from build123d import *

# Parameters (mm, degrees)
F0_W     = 119.99976
F0_H     = 125.00102
F1_DEPTH = 10
F2_W     = 12.7
F2_H     = 25.4
F3_DEPTH = 2.54
F4_R     = 6.35
F5_DEPTH = 7.62
F6_R     = 1.27
F7_R     = 2.54
F8_R     = 2.54
F9_DEPTH = 125.00202
F10_R    = 2.54


with BuildPart() as f1:
    # F0 (on Top) → F1 (new body)
    with BuildSketch(Plane.XY):
        Rectangle(F0_W, F0_H)
    extrude(amount=F1_DEPTH)

    # F2 (on face) → F3 (cut)
    with BuildSketch(Plane.XY.offset(10)):
        with Locations((53.64988, -37.59327)):
            Rectangle(F2_W, F2_H)
        Polygon((47.29988, -12.7), (59.99988, -12.7), (59.99988, 12.7), (47.29988, 12.7), (47.29988, 0), align=None)
        with Locations((53.64988, 37.59327)):
            Rectangle(F2_W, F2_H)
    extrude(amount=-F3_DEPTH, mode=Mode.SUBTRACT)

    # F4 (on face) → F5 (join)
    with BuildSketch(Plane.XY.offset(10)):
        with Locations((-40.94988, 0)):
            Circle(F4_R)
        with Locations((-40.94988, -31.24962)):
            Circle(F4_R)
        with Locations((-40.94988, 31.24962)):
            Circle(F4_R)
    extrude(amount=F5_DEPTH)

    # F6
    f6_edges = [f1.edges().sort_by_distance(p)[0] for p in [
        (-47.29988, -31.24962, 17.62),
        (-47.29988, 0, 17.62),
        (-47.29988, 31.24962, 17.62),
    ]]
    fillet(f6_edges, radius=F6_R)

    # F7
    f7_edges = [f1.edges().sort_by_distance(p)[0] for p in [
        (-59.99988, 62.50051, 5),
        (-59.99988, -62.50051, 5),
        (0, 62.50051, 0),
        (-59.99988, 0, 0),
        (0, -62.50051, 0),
        (59.99988, 0, 0),
    ]]
    fillet(f7_edges, radius=F7_R)

    # F8 (on face) → F9 (cut, through all)
    with BuildSketch(Plane.XZ.offset(62.50051)):
        with Locations((59.99988, 10)):
            Circle(F8_R)
    extrude(amount=-F9_DEPTH, mode=Mode.SUBTRACT)

    # F10
    f10_edges = [f1.edges().sort_by_distance(p)[0] for p in [
        (57.45988, 56.39689, 10),
        (57.45988, 18.796635, 10),
        (57.45988, -18.796635, 10),
        (57.45988, -56.39689, 10),
    ]]
    fillet(f10_edges, radius=F10_R)


solid = f1.part
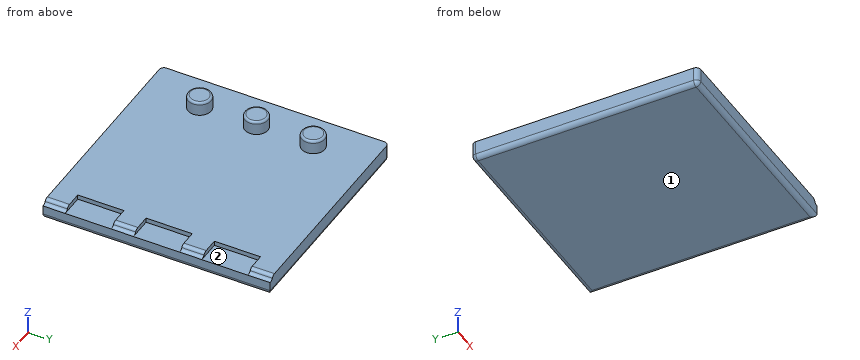
CAD build for the part. Positions are in the model's coordinates, mm. Face numbers are marked on the shaded views. A direction names the side the tool comes from. Coordinates: 2 decimals unless noted, no trailing zeros. Loops run counter-clockwise (first coordinate to the right, second up) from the corner with the lowest first, then second, coordinate; pieces in that order, holes last. Notation, with made-up numbers: (-12, 63.5) -> (-2, 63.5) arc R7 cw to (-2, 69.5) -> close; hole circle Ø1 at (-6.75, 87). An arc over 180 degrees is marked (long way). One line per item, written item: value.
1. Slice it at C-C on z = 14.25. Write the cut outline in (x, y), and give its area (3 significant figures).
Answers:
outline: circle Ø12.7 at (-40.95, -31.25); circle Ø12.7 at (-40.95, 0); circle Ø12.7 at (-40.95, 31.25)
area: 380 mm^2
2. Flat gauge pins, fed straight in: P1, Ø3, axis at y = -3, z = 9, coming from the +X side; P2, Ø6.5, axis at x = 51, y = 32, coming from the +Z side; P3, Ø10, axis at y = 40, z = 15.5, coming from the +X side. Where does each tip first touch, or does it go through?
Answers:
P1: stops at x = 47.3
P2: stops at z = 7.46
P3: stops at x = -35.83
3. Which spindle directions (+Z, -Z, +X, -X, +Y, -Y) get a long thin tool onto all of the face, cutting with end or side? Do the marked faces 1 and 2. Say none if no direction does.
Answers:
face 1: -Z, +X, -X, +Y, -Y
face 2: +Z, +X
4. Drill centre lines: line 1 (X direction, y = -39, z = 7.5); line 2 (Z direction, x = 17.5, y = 0.5); line 3 (X direction, y = 19, z = 2.25). Where is each one in solid material? Low to high. Write a range as [from, to].
Answers:
line 1: x = [-60, 47.3]
line 2: z = [0, 10]
line 3: x = [-59.98, 59.98]
5. Slice it at B-B on y = 53.5. Write the cut outline in (x, z).
Answers:
outline: (-60, 2.54) arc R2.54 ccw to (-57.46, 0) -> (57.46, 0) arc R2.54 ccw to (60, 2.54) -> (60, 7.46) arc R2.54 cw to (57.8, 8.73) arc R2.54 ccw to (55.6, 10) -> (-60, 10) -> close
6. Slice it at D-D on y = 0. Write the cut outline in (x, z), and give its area (3 significant figures).
Answers:
outline: (-60, 2.54) arc R2.54 ccw to (-57.46, 0) -> (57.46, 0) arc R2.54 ccw to (60, 2.54) -> (60, 7.46) -> (47.3, 7.46) -> (47.3, 10) -> (-34.6, 10) -> (-34.6, 16.35) arc R1.27 ccw to (-35.87, 17.62) -> (-46.03, 17.62) arc R1.27 ccw to (-47.3, 16.35) -> (-47.3, 10) -> (-60, 10) -> close
area: 1,260 mm^2
7. Slice it at A-A on x = -24. Write the cut outline in (y, z), and give its area (3 significant figures).
Answers:
outline: (-62.5, 2.54) arc R2.54 ccw to (-59.96, 0) -> (59.96, 0) arc R2.54 ccw to (62.5, 2.54) -> (62.5, 10) -> (-62.5, 10) -> close
area: 1,250 mm^2
